Here's the drawing with two shaded views (mm, measured from the low corner). I have some questions. A direction names the side the tool comes from. Give positions to 0.01 mm unless a question says otherwise; leave off trailing zeros. Loops run counter-clockwise (first coordinate to the right, second up) from the corner with the lowest first, then second, coordinate; pieces in that order, holes last. Notation, with made-up numbers: (53.5, 21) -> (60.5, 21) arc R9 ccw to (60.5, 27) -> close; hole circle Ø4 at (43, 33). An arc over 180 degrees is marked (long way). Write each question's results on one line, items separated by ' | '. Start each with the question number.
Q1. Which directions (+Z, -Z, +X, -X, +Y, -Y) give clear straight access to the entire face, cutting with the end or side of a thin tool? Please do the marked faces 1 and 2.
Q2. Will these pins go through, and if not, where does the flat tip stop? P1, Ø6.5, axis at y = 3, z = 38, coming from the +X side; P2, Ø10.5, axis at x = 37.5, z = 45, coming from the -Y side; P3, Ø4, axis at x = 37.5, z = 57, coming from the -Y side; P4, Ø1, axis at x = 55, z = 79.5, coming from the -Y side.
Q3. If we section it at D-D, the plane z = 16.5: List the corners of the cut face in (x, y) for me.
Q4. If I drill on line 1 along Z through (x, y) = (37, 5); line 2 along Y through (x, z) = (32, 36); line 3 along Z through (x, y) = (49.5, 3), over which ranges is the centre line in solid material (lowest first)?
Q5. If we section it at A-A, the plane x = 37.5: List the corners of the cut face in (y, z) for me, plus the area to 3 significant figures.
Q6. If we section it at C-C, the plane y = 28.5: List the corners of the cut face in (x, z) for me.
Q7. We'd pull the mould along Z, two halves only. Please class the marked faces 3, 4 and 5: released by +Z, released by -Z, zero draft, split by the parting line, or undercut.
Q8. If we section it at B-B, the plane z = 57: List the corners of the cut face in (x, y) for me.
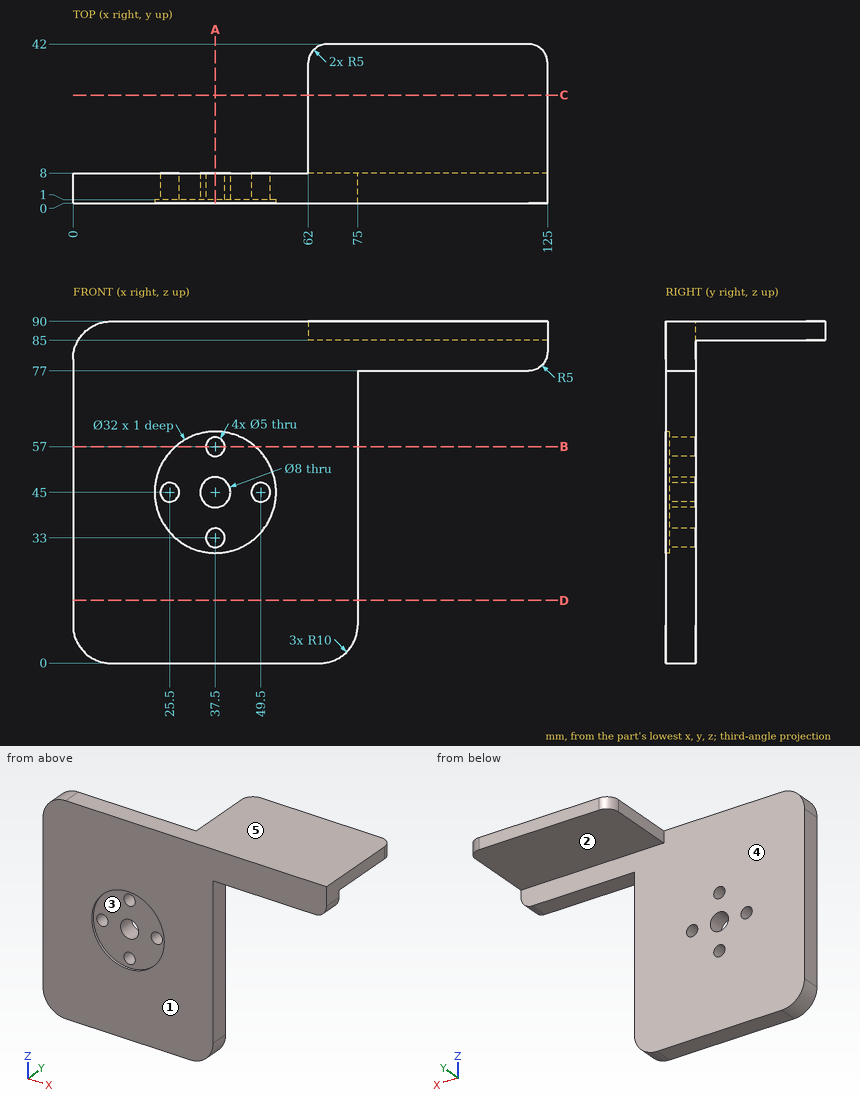
Final values:
1) face 1: +Z, -Z, +X, -X, -Y | face 2: -Z, +X, -X, +Y
2) P1: stops at x = 75 | P2: stops at y = 1 | P3: passes through | P4: stops at y = 0
3) outline: (0, 0) -> (75, 0) -> (75, 8) -> (0, 8) -> close
4) line 1: z = 0 to 30.55, 35.45 to 41.03, 48.97 to 54.55, 59.45 to 90 | line 2: y = 1 to 8 | line 3: z = 0 to 42.5, 47.5 to 90
5) outline: (0, 0) -> (8, 0) -> (8, 30.5) -> (1, 30.5) -> (1, 29) -> (0, 29) -> close; (0, 61) -> (1, 61) -> (1, 59.5) -> (8, 59.5) -> (8, 90) -> (0, 90) -> close; (1, 35.5) -> (8, 35.5) -> (8, 41) -> (1, 41) -> close; (1, 49) -> (8, 49) -> (8, 54.5) -> (1, 54.5) -> close | area: 562 mm²
6) outline: (62, 85) -> (125, 85) -> (125, 90) -> (62, 90) -> close
7) face 3: undercut | face 4: zero draft | face 5: released by +Z
8) outline: (0, 0) -> (26.92, 0) -> (26.92, 1) -> (35, 1) -> (35, 8) -> (0, 8) -> close; (40, 1) -> (48.08, 1) -> (48.08, 0) -> (75, 0) -> (75, 8) -> (40, 8) -> close
